Work out the finished part from the listing and answer in its coordinate system (mm). A direction names the side the tool comes from. Give positions to 0.01 mm unless a question says otherwise; leave off trailing zeros. Loops run counter-clockwise (first coordinate to the right, second up) from the corner with the lowest first, then second, coordinate; pieces in that order, holes last. Notation, with made-up numbers: M -31,58 L 24,58 A36 ccw 24,97 Z; hole C 3,75 d7. An arc over 180 degrees is marked long. Use a Markdown table: item, result.
```python
from build123d import *

# Parameters (mm, degrees)
SKETCH1_R                   = 75
SKETCH1_R_2                 = 28
BOSS_EXTRUDE1_DEPTH         = 3
CUT_EXTRUDE2_START          = -3
CUT_EXTRUDE2_DEPTH          = 3
CIRPATTERN1_COUNT           = 4
TAP_DRILL_FOR_M4X0_7_TAP1_D = 3.3
CIRPATTERN2_COUNT           = 4


with BuildPart() as part:
    # Sketch1 → Boss-Extrude1 (new body)
    with BuildSketch(Plane(origin=(0, 0, 0), x_dir=(1, 0, 0), z_dir=(0, 1, 0))):
        with Locations(Location((0, 0, 0), (0, 0, 270))):
            Circle(SKETCH1_R)
        with Locations(Location((0, 0, 0), (0, 0, 270))):
            Circle(SKETCH1_R_2, mode=Mode.SUBTRACT)
    extrude(amount=BOSS_EXTRUDE1_DEPTH)

    # Sketch2 → Cut-Extrude2 (cut)
    with BuildSketch(Plane(origin=(0, 3, 0), x_dir=(1, 0, 0), z_dir=(0, 1, 0)).offset(CUT_EXTRUDE2_START)):
        with BuildLine():
            Line((5.5, 27.454507827), (5.5, 48))
            ThreePointArc((5.5, 48), (0, 53.5), (-5.5, 48))
            Line((-5.5, 48), (-5.5, 27.454507827))
            ThreePointArc((-5.5, 27.454507827), (0, 28), (5.5, 27.454507827))
        make_face()
    cut_extrude2 = extrude(amount=CUT_EXTRUDE2_DEPTH, mode=Mode.SUBTRACT)

    # CirPattern1: Cut-Extrude2 ×4 about axis
    cirpattern1_axis = Axis((0, 0, 0), (0, 1, 0))
    for i in range(1, CIRPATTERN1_COUNT):
        add(cut_extrude2.rotate(cirpattern1_axis, i * 360 / CIRPATTERN1_COUNT), mode=Mode.SUBTRACT)

    # Tap Drill for M4x0.7 Tap1 (through all)
    with Locations(Plane(origin=(0, 3, 0), x_dir=(1, 0, 0), z_dir=(0, 1, 0))):
        with Locations((38, 38)):
            tap_drill_for_m4x0_7_tap1 = Hole(TAP_DRILL_FOR_M4X0_7_TAP1_D / 2)

    # CirPattern2: Tap Drill for M4x0.7 Tap1 ×4 about axis
    cirpattern2_axis = Axis((0, 0, 0), (0, 1, 0))
    for i in range(1, CIRPATTERN2_COUNT):
        add(tap_drill_for_m4x0_7_tap1.rotate(cirpattern2_axis, i * 360 / CIRPATTERN2_COUNT), mode=Mode.SUBTRACT)


solid = part.part
```
(1) Which of the six approach directions +Z, -Z, +X, -X, +Y, -Y give full straight-line access (tool end or side, diameter ignored) to faces 1 (the cylindrical face through (-19.961, 1.479, 19.635)), 2 (the flat face through (-32, 0, 16))?
Entries:
| item | result |
|---|---|
| face 1 | +Y, -Y |
| face 2 | +Z, -Z, +X, -X, -Y |
(2) Consider probe 1 along Z at (x, y) = (38, 1.35); probe 2 along X at (y, z) = (0.85, -36). Determine where each line is inside the solid, lowest interval first. Write a range as [from, to].
Entries:
| item | result |
|---|---|
| probe 1 | z = [-64.66, -39.65], [-36.35, -5.5], [5.5, 36.35], [39.65, 64.66] |
| probe 2 | x = [-65.8, -5.5], [5.5, 65.8] |
(3) Given P1, Ø2.5, axis at x = 38, z = -38, coming from the +Y side; P2, Ø0.9, axis at x = 36, y = 2, coming from the +Z side; P3, Ø0.9, axis at x = -35.5, y = 1.5, coming from the +Z side; P4, Ø1.5, axis at x = -34.5, y = 1.5, coming from the -Z side, each flat-ended and moving along its own axis, determine where each tip first touches the part or whether it passes through.
Entries:
| item | result |
|---|---|
| P1 | passes through |
| P2 | stops at z = 66.04 |
| P3 | stops at z = 66.31 |
| P4 | stops at z = -66.98 |
(4) A cutting plane is placed at D-D (x = -61). Write down the section's boundary in (y, z), and give its area (3 significant figures).
Entries:
| item | result |
|---|---|
| outline | M 0,-43.63 L 3,-43.63 L 3,43.63 L 0,43.63 Z |
| area | 262 mm² |
(5) The mould has two halves that part along X. Classify faces 3 (the cylindrical face through (39.216, 1.479, -39.115)), 4 (the flat face through (-32, 3, 16)), 5 (the cylindrical face through (-45.636, 1.479, -59.517)): released by +X, released by -X, zero draft, split by the parting line, or undercut.
Entries:
| item | result |
|---|---|
| face 3 | undercut |
| face 4 | zero draft |
| face 5 | split by the parting line |
(6) A cutting plane is placed at B-B (x = 0). Write down the section's boundary in (y, z).
Entries:
| item | result |
|---|---|
| outline | M 0,-75 L 3,-75 L 3,-53.5 L 0,-53.5 Z; M 0,53.5 L 3,53.5 L 3,75 L 0,75 Z |
(7) A cutting plane is placed at C-C (y = 1.5). Write down the section's boundary in (x, z), and give its area (3 significant figures).
Entries:
| item | result |
|---|---|
| outline | C 0,0 d150; hole M -48,-5.5 L -27.45,-5.5 A28 ccw -5.5,-27.45 L -5.5,-48 A5.5 ccw 5.5,-48 L 5.5,-27.45 A28 ccw 27.45,-5.5 L 48,-5.5 A5.5 ccw 48,5.5 L 27.45,5.5 A28 ccw 5.5,27.45 L 5.5,48 A5.5 ccw -5.5,48 L -5.5,27.45 A28 ccw -27.45,5.5 L -48,5.5 A5.5 ccw Z; hole C -38,-38 d3.3; hole C -38,38 d3.3; hole C 38,-38 d3.3; hole C 38,38 d3.3 |
| area | 14,100 mm² |
(8) A cutting plane is placed at A-A (z = 0). Write down the section's boundary in (x, y).
Entries:
| item | result |
|---|---|
| outline | M -75,0 L -53.5,0 L -53.5,3 L -75,3 Z; M 53.5,0 L 75,0 L 75,3 L 53.5,3 Z |
